Source: CAD feature listing. Evaluate the final solid. Frame: model axes, mm. A direction names the side the tool comes from. Round coordinates to 2 decimals unless told otherwise and drop trailing zeros. Order: outer loops, then holes, each group sorted by start corner. A loop starts at its lowest first (then second) coordinate and runs counter-clockwise, first axis right, second up. Notation, with made-up numbers: (57.25, -1) -> (115.25, -1) arc R7 ccw to (115.25, 8) -> close; hole circle Ø11 at (61, 33). An arc over 180 degrees is marked (long way). Answer as CSV lines item,"result". Start each with the question number.
(1) Pull-direction query (Z, two-part tool) for faces 1 (the flat face through (-2.5, -16, 59)), 2 (the flat face through (-46, 0, 61)), 3 (the flat face through (-46, -15, 120)); classes: +Z half, -Z half, draft (parallel to the pull), parting line (faces both ways), or undercut.
(2) Section query B-B (x = -10.5). Output: boundary loops of the cut face in (y, z).
(3) Section query C-C (z = 79). Output: boundary loops of the cut face in (x, y).
(4) Line query: line 1 along X through (y, z) = (-24, 38); line 2 along Z through (x, y) = (-62, -27.75); line 3 along Y through (x, z) = (-57, 105). Output: solid intervals per line, ascending. Write a range as from..to.
(5) Section query A-A (y = -6.5). Output: boundary loops of the cut face in (x, z).
(6) Set-up query: faces 4 (the flat face through (-45, -30, 118)), 5 (the flat face through (-46, -2.5, 61)). Return all of +Z, -Z, +X, -X, +Y, -Y with unobstructed straight access to the full face (end or side cutting, diameter ignored); none if empty.
```python
from build123d import *

# Parameters (mm, degrees)
F0_W     = 90
F0_H     = 120
F1_DEPTH = 30
F2_T     = -2.5
F3_R     = 1
F4_DEPTH = 120.001


with BuildPart() as f1:
    # F0 (on Front) → F1 (new body)
    with BuildSketch(Plane.XZ):
        with Locations((-45, 60)):
            Rectangle(F0_W, F0_H)
    extrude(amount=F1_DEPTH)

    # F2
    f2_openings = [f1.faces().sort_by_distance(p)[0] for p in [
        (-45, -30, 60),
    ]]
    offset(amount=F2_T, openings=f2_openings)

    # F3 (on face) → F4 (cut, through all)
    with BuildSketch(Plane.XY.offset(120)):
        with Locations((-47.093008, -12.78865)):
            Circle(F3_R)
    extrude(amount=-F4_DEPTH, mode=Mode.SUBTRACT)


solid = f1.part
```
Answer block:
1,face 1,"undercut"
1,face 2,"draft"
1,face 3,"+Z half"
2,outline,"(-30, 0) -> (0, 0) -> (0, 120) -> (-30, 120) -> (-30, 117.5) -> (-2.5, 117.5) -> (-2.5, 2.5) -> (-30, 2.5) -> close"
3,outline,"(-90, -30) -> (-87.5, -30) -> (-87.5, -2.5) -> (-2.5, -2.5) -> (-2.5, -30) -> (0, -30) -> (0, 0) -> (-90, 0) -> close"
4,line 1,"-90..-87.5, -2.5..0"
4,line 2,"0..2.5, 117.5..120"
4,line 3,"-2.5..0"
5,outline,"(-90, 0) -> (0, 0) -> (0, 120) -> (-90, 120) -> close; hole (-87.5, 2.5) -> (-2.5, 2.5) -> (-2.5, 117.5) -> (-87.5, 117.5) -> close"
6,face 4,"+Z, -Z, +X, -X, -Y"
6,face 5,"-Y"
